```python
from build123d import *

# Parameters (mm, degrees)
SKIZZE1_W                        = 65
SKIZZE1_H                        = 160
AUFSATZ_LINEAR_AUSTRAGEN1_DEPTH  = 10
SKIZZE2_R                        = 16
SCHNITT_LINEAR_AUSTRAGEN1_DEPTH  = 8
SKIZZE3_W                        = 20
SKIZZE3_H                        = 3
SCHNITT_LINEAR_AUSTRAGEN2_DEPTH  = 15
SKIZZE4_R                        = 4
SCHNITT_LINEAR_AUSTRAGEN3_DEPTH  = 20
SKIZZE6_R                        = 14
SCHNITT_LINEAR_AUSTRAGEN4_DEPTH  = 20
SKIZZE7_R                        = 1.62
SCHNITT_LINEAR_AUSTRAGEN5_DEPTH  = 5
SKIZZE8_R                        = 1.62
SCHNITT_LINEAR_AUSTRAGEN6_DEPTH  = 5
SKIZZE9_R                        = 3
SCHNITT_LINEAR_AUSTRAGEN7_DEPTH  = 32
FASE1_SIZE                       = 3.3
SKIZZE10_R                       = 3
SCHNITT_LINEAR_AUSTRAGEN8_DEPTH  = 32
FASE2_SIZE                       = 3.3
SKIZZE11_R                       = 3
SCHNITT_LINEAR_AUSTRAGEN9_DEPTH  = 32
FASE3_SIZE                       = 3.3
SKIZZE12_R                       = 3
SCHNITT_LINEAR_AUSTRAGEN10_DEPTH = 25
FASE4_SIZE                       = 3.3
SKIZZE13_W                       = 10
SKIZZE13_H                       = 160
SCHNITT_LINEAR_AUSTRAGEN11_DEPTH = 5


with BuildPart() as part:
    # Skizze1 → Aufsatz-Linear austragen1 (new body)
    with BuildSketch(Plane.XY):
        with Locations((32.5, 80)):
            Rectangle(SKIZZE1_W, SKIZZE1_H)
    extrude(amount=AUFSATZ_LINEAR_AUSTRAGEN1_DEPTH)

    # Skizze2 → Schnitt-Linear austragen1 (cut)
    with BuildSketch(Plane(origin=(0, 0, 0), x_dir=(-1, 0, 0), z_dir=(0, 0, -1))):
        with Locations((-21.15, 80)):
            Circle(SKIZZE2_R)
    extrude(amount=-SCHNITT_LINEAR_AUSTRAGEN1_DEPTH, mode=Mode.SUBTRACT)

    # Skizze3 → Schnitt-Linear austragen2 (cut)
    with BuildSketch(Plane(origin=(0, 160, 0), x_dir=(1, 0, 0), z_dir=(0, 1, 0))):
        with Locations((10, -1.5)):
            Rectangle(SKIZZE3_W, SKIZZE3_H)
    extrude(amount=-SCHNITT_LINEAR_AUSTRAGEN2_DEPTH, mode=Mode.SUBTRACT)

    # Skizze4 → Schnitt-Linear austragen3 (cut)
    with BuildSketch(Plane(origin=(0, 0, 0), x_dir=(-1, 0, 0), z_dir=(0, 0, -1))):
        with Locations((-21.15, 130)):
            Circle(SKIZZE4_R)
    extrude(amount=-SCHNITT_LINEAR_AUSTRAGEN3_DEPTH, mode=Mode.SUBTRACT)

    # Skizze6 → Schnitt-Linear austragen4 (cut)
    with BuildSketch(Plane(origin=(0, 0, 8), x_dir=(-1, 0, 0), z_dir=(0, 0, -1))):
        with Locations((-21.15, 80)):
            Circle(SKIZZE6_R)
    extrude(amount=-SCHNITT_LINEAR_AUSTRAGEN4_DEPTH, mode=Mode.SUBTRACT)

    # Skizze7 → Schnitt-Linear austragen5 (cut)
    with BuildSketch(Plane(origin=(0, 0, 3), x_dir=(-1, 0, 0), z_dir=(0, 0, -1))):
        with Locations((-5, 151)):
            Circle(SKIZZE7_R)
    extrude(amount=-SCHNITT_LINEAR_AUSTRAGEN5_DEPTH, mode=Mode.SUBTRACT)

    # Skizze8 → Schnitt-Linear austragen6 (cut)
    with BuildSketch(Plane(origin=(0, 0, 3), x_dir=(-1, 0, 0), z_dir=(0, 0, -1))):
        with Locations((-15, 151)):
            Circle(SKIZZE8_R)
    extrude(amount=-SCHNITT_LINEAR_AUSTRAGEN6_DEPTH, mode=Mode.SUBTRACT)

    # Skizze9 → Schnitt-Linear austragen7 (cut)
    with BuildSketch(Plane.XY.offset(10)):
        with Locations((15, 12)):
            Circle(SKIZZE9_R)
    extrude(amount=-SCHNITT_LINEAR_AUSTRAGEN7_DEPTH, mode=Mode.SUBTRACT)

    # Fase1
    fase1_edges = [part.edges().sort_by_distance(p)[0] for p in [
        (12, 12, 10),
    ]]
    chamfer(fase1_edges, length=FASE1_SIZE)

    # Skizze10 → Schnitt-Linear austragen8 (cut)
    with BuildSketch(Plane.XY.offset(10)):
        with Locations((50, 12)):
            Circle(SKIZZE10_R)
    extrude(amount=-SCHNITT_LINEAR_AUSTRAGEN8_DEPTH, mode=Mode.SUBTRACT)

    # Fase2
    fase2_edges = [part.edges().sort_by_distance(p)[0] for p in [
        (47, 12, 10),
    ]]
    chamfer(fase2_edges, length=FASE2_SIZE)

    # Skizze11 → Schnitt-Linear austragen9 (cut)
    with BuildSketch(Plane.XY.offset(10)):
        with Locations((15, 30)):
            Circle(SKIZZE11_R)
    extrude(amount=-SCHNITT_LINEAR_AUSTRAGEN9_DEPTH, mode=Mode.SUBTRACT)

    # Fase3
    fase3_edges = [part.edges().sort_by_distance(p)[0] for p in [
        (12, 30, 10),
    ]]
    chamfer(fase3_edges, length=FASE3_SIZE)

    # Skizze12 → Schnitt-Linear austragen10 (cut)
    with BuildSketch(Plane.XY.offset(10)):
        with Locations((50, 30)):
            Circle(SKIZZE12_R)
    extrude(amount=-SCHNITT_LINEAR_AUSTRAGEN10_DEPTH, mode=Mode.SUBTRACT)

    # Fase4
    fase4_edges = [part.edges().sort_by_distance(p)[0] for p in [
        (47, 30, 10),
    ]]
    chamfer(fase4_edges, length=FASE4_SIZE)

    # Skizze13 → Schnitt-Linear austragen11 (cut)
    with BuildSketch(Plane(origin=(65, 0, 0), x_dir=(0, 0, -1), z_dir=(1, 0, 0))):
        with Locations((-5, 80)):
            Rectangle(SKIZZE13_W, SKIZZE13_H)
    extrude(amount=-SCHNITT_LINEAR_AUSTRAGEN11_DEPTH, mode=Mode.SUBTRACT)


solid = part.part
```
Verification items for the finished model (mm, model axes). A direction names the side the tool comes from. Round coordinates to 2 decimals unless told otherwise and drop trailing zeros. Write each loop counter-clockwise with the first axis right and the second up, starting at its lowest first coordinate (ties: lowest second). Pieces come first, ordered by that corner, then holes. Notation, with made-up numbers: (73.25, -8) -> (114.25, -8) arc R25 ccw to (114.25, 12) -> close; hole circle Ø2 at (-8.5, -30). An arc over 180 degrees is marked (long way). Write each question's results on one line, items separated by ' | '. Start each with the question number.
1. Material ranges on probe 1 along Y at (x, z) = (21.15, 6); probe 2 along Y at (x, z) = (18.5, 3.5); probe 3 along Y at (x, z) = (15, 3.5), recorded low to high. Write a range as from..to.
2. Cross-section at C-C (z = 4.5). Count the separate pieces of the cut face and the enclosed holes in it, then the cut area to 3 significant figures.
3. Cross-section at B-B (y = 130). Enter the section's corners in (x, z), then the cut area to 3 significant figures.
4. Cross-section at D-D (y = 151). Enter the section's corners in (x, z).
5. Draft check along Y on faces 4 (the flat face through (43, 81, 0)), 5 (the cylindrical face through (15.35, 149.42, 5.46)), 6 (the flat face through (30, 0, 5)). Enter one of: +Y half, -Y half, draft (parallel to the pull), parting line (faces both ways), or undercut.
6. Depth check by flat-ended pin: P1, Ø3.5, axis at x = 15, y = 150.5, coming from the -Z side; P2, Ø0.9, axis at x = 12, z = 1.5, coming from the +Y side; P3, Ø1.6, axis at x = 5.5, y = 151.5, coming from the -Z side. Enter the tip coordinate at first touch or a pass-through.
7. Cross-section at A-A (y = 12). Enter the section's corners in (x, z).
8. Set-up check for faces 1 (the flat face through (5, 151, 8)), 2 (the flat face through (10, 153, 3)), 3 (the cylindrical face through (12.6, 10.2, 3.4)): record each of +Z, -Z, +X, -X, +Y, -Y from which the full face is reachable in a straight line by a thin tool's end or side.
Solutions:
1) probe 1: y = 0..64, 96..126, 134..160 | probe 2: y = 0..64.22, 95.78..127, 133..160 | probe 3: y = 0..9, 15..27, 33..65.23, 94.77..149.38, 152.62..160
2) separate pieces: 1 | enclosed holes: 8 | area: 8,620 mm2
3) outline: (0, 0) -> (17.15, 0) -> (17.15, 10) -> (0, 10) -> close; (25.15, 0) -> (60, 0) -> (60, 10) -> (25.15, 10) -> close | area: 520 mm2
4) outline: (0, 3) -> (3.38, 3) -> (3.38, 8) -> (6.62, 8) -> (6.62, 3) -> (13.38, 3) -> (13.38, 8) -> (16.62, 8) -> (16.62, 3) -> (20, 3) -> (20, 0) -> (60, 0) -> (60, 10) -> (0, 10) -> close
5) face 4: draft | face 5: undercut | face 6: -Y half
6) P1: stops at z = 3 | P2: stops at y = 145 | P3: stops at z = 8
7) outline: (0, 0) -> (12, 0) -> (12, 6.7) -> (8.7, 10) -> (0, 10) -> close; (18, 0) -> (47, 0) -> (47, 6.7) -> (43.7, 10) -> (21.3, 10) -> (18, 6.7) -> close; (53, 0) -> (60, 0) -> (60, 10) -> (56.3, 10) -> (53, 6.7) -> close
8) face 1: -Z | face 2: -Z, -X, +Y | face 3: +Z, -Z
